Part model, mm, in its own coordinate system. Face numbers are marked on the shaded views. Give positions to 0.01 mm unless a question says otherwise; leave off trailing zeros. Order: outer loops, then holes, each group sorted by start corner. A loop starts at its lowest first (then second) coordinate and runs counter-clockwise, first axis right, second up. Notation, with made-up numbers: (20.25, -3.5) - (67.25, -3.5) arc R16 cw to (67.25, 3.5) - close; hole circle Ø1 at (82, 3). An arc over 180 degrees is marked (long way). One line per item, written item: value.
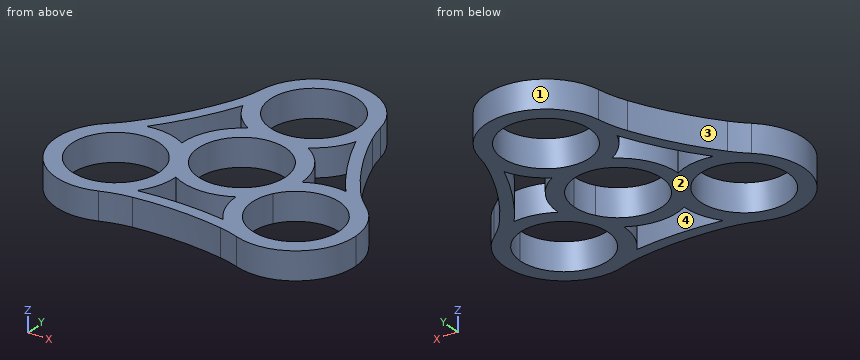
```python
from build123d import *

# Parameters (mm, degrees)
F1_DEPTH = 7
F2_R     = 30


with BuildPart() as f1:
    # F0 (on Top) → F1 (new body)
    with BuildSketch(Plane.XY):
        with BuildLine():
            ThreePointArc((-13.9458281821, 20.4760633317), (-11.3479038896, 16.1905618249), (-7.4833147735, 13))
            ThreePointArc((-7.4833147735, 13), (-3.8729833256, 14.4913767517), (4.26e-08, 15))
            ThreePointArc((4.26e-08, 15), (3.8729833668, 14.4913767407), (7.4833147735, 13))
            ThreePointArc((7.4833147735, 13), (11.4579364901, 16.3193134856), (14.0670033826, 20.7923694606))
            ThreePointArc((14.0670033826, 20.7923694606), (14.7649085798, 23.3547259819), (15, 26))
            ThreePointArc((15, 26), (14.9881318268, 26.5965771885), (14.9525460877, 27.1922103396))
            ThreePointArc((14.9525460877, 27.1922103396), (-0.6061990993, 40.9877457495), (-14.999987636, 25.9807406984))
            ThreePointArc((-14.999987636, 25.9807406984), (-14.7322921357, 23.1787292883), (-13.9458281821, 20.4760633317))
        make_face()
        with BuildLine():
            ThreePointArc((11, 26), (7.7781746081, 18.221825422), (4.26e-08, 15))
            ThreePointArc((4.26e-08, 15), (-7.7781746081, 33.778174578), (11, 26))
        make_face(mode=Mode.SUBTRACT)
        with BuildLine():
            ThreePointArc((-7.4833147735, 13), (-3.8729833208, 11.508623247), (5.26e-08, 11))
            ThreePointArc((5.26e-08, 11), (3.8729833716, 11.5086232606), (7.4833147735, 13))
            ThreePointArc((7.4833147735, 13), (3.8729833668, 14.4913767407), (4.26e-08, 15))
            ThreePointArc((4.26e-08, 15), (-3.8729833256, 14.4913767517), (-7.4833147735, 13))
        make_face()
        with BuildLine():
            ThreePointArc((5.26e-08, 11), (7.7781746116, 7.7781745745), (11, 0))
            ThreePointArc((11, 0), (10.6251840814, -2.8470095251), (9.5262794117, -5.5000000519))
            ThreePointArc((9.5262794117, -5.5000000519), (11.9032517523, -2.4002096819), (14.999987636, -0.0192593016))
            ThreePointArc((14.999987636, -0.0192593016), (14.999996909, -0.0096296528), (15, 0))
            ThreePointArc((15, 0), (12.9855635535, 7.5083379784), (7.4833147735, 13))
            ThreePointArc((7.4833147735, 13), (3.8729833716, 11.5086232606), (5.26e-08, 11))
        make_face()
        with BuildLine():
            ThreePointArc((15, 26), (14.7649085798, 23.3547259819), (14.0670033826, 20.7923694606))
            ThreePointArc((14.0670033826, 20.7923694606), (18.7632858244, 10.9661480048), (24.7057051058, 1.8394098167))
            ThreePointArc((24.7057051058, 1.8394098167), (27.439514459, 1.1691746013), (29.9999752719, 0))
            ThreePointArc((29.9999752719, 0), (21.1431293427, 12.8583865681), (14.9525460877, 27.1922103396))
            ThreePointArc((14.9525460877, 27.1922103396), (14.9881318268, 26.5965771885), (15, 26))
        make_face()
        with BuildLine():
            ThreePointArc((24.7057051058, 1.8394098167), (19.6953897867, 1.7322921357), (14.999987636, -0.0192593016))
            ThreePointArc((14.999987636, -0.0192593016), (14.4863920627, -3.8915864381), (12.9903810244, -7.5000000561))
            ThreePointArc((12.9903810244, -7.5000000561), (10.613408702, -10.5997903623), (7.5166728624, -12.9807406984))
            ThreePointArc((7.5166728624, -12.9807406984), (8.4039718058, -18.0825208181), (10.9732184665, -22.5785670147))
            ThreePointArc((10.9732184665, -22.5785670147), (13.3069353398, -24.8398041582), (16.0728718952, -26.545389933))
            ThreePointArc((16.0728718952, -26.545389933), (30.5273774124, -25.681814323), (37.5166604984, -13))
            ThreePointArc((37.5166604984, -13), (35.5022240519, -5.4916620216), (29.9999752719, 0))
            ThreePointArc((29.9999752719, 0), (27.439514459, 1.1691746013), (24.7057051058, 1.8394098167))
        make_face()
        with BuildLine():
            ThreePointArc((33.5166604984, -13), (19.6696510336, -23.6251840976), (12.9903810244, -7.5000000561))
            ThreePointArc((12.9903810244, -7.5000000561), (25.3636699632, -2.3748159024), (33.5166604984, -13))
        make_face(mode=Mode.SUBTRACT)
        with BuildLine():
            ThreePointArc((14.999987636, -0.0192593016), (11.9032517523, -2.4002096819), (9.5262794117, -5.5000000519))
            ThreePointArc((9.5262794117, -5.5000000519), (8.0302684195, -9.1084136221), (7.5166728624, -12.9807406984))
            ThreePointArc((7.5166728624, -12.9807406984), (10.613408702, -10.5997903623), (12.9903810244, -7.5000000561))
            ThreePointArc((12.9903810244, -7.5000000561), (14.4863920627, -3.8915864381), (14.999987636, -0.0192593016))
        make_face()
        with BuildLine():
            ThreePointArc((7.5166728624, -12.9807406984), (8.0302684195, -9.1084136221), (9.5262794117, -5.5000000519))
            ThreePointArc((9.5262794117, -5.5000000519), (-5.2e-09, -11), (-9.5262794169, -5.5000000429))
            ThreePointArc((-9.5262794169, -5.5000000429), (-8.0302684209, -9.1084136171), (-7.5166728624, -12.9807406984))
            ThreePointArc((-7.5166728624, -12.9807406984), (0, -15), (7.5166728624, -12.9807406984))
        make_face()
        with BuildLine():
            ThreePointArc((16.0728718952, -26.545389933), (13.3069353398, -24.8398041582), (10.9732184665, -22.5785670147))
            ThreePointArc((10.9732184665, -22.5785670147), (0.1153198416, -21.7325561849), (-10.7598769237, -22.3154731484))
            ThreePointArc((-10.7598769237, -22.3154731484), (-12.7072223233, -24.3479038896), (-14.999987636, -25.9807406984))
            ThreePointArc((-14.999987636, -25.9807406984), (0.5641247483, -24.7396804103), (16.0728718952, -26.545389933))
        make_face()
        with BuildLine():
            ThreePointArc((-7.5166604984, -13), (-7.5166635894, -12.9903703472), (-7.5166728624, -12.9807406984))
            ThreePointArc((-7.5166728624, -12.9807406984), (-10.6134087435, -10.5997903208), (-12.990381083, -7.4999999545))
            ThreePointArc((-12.990381083, -7.4999999545), (-14.4863920779, -3.8915863815), (-14.999987636, -0.0192593016))
            ThreePointArc((-14.999987636, -0.0192593016), (-19.8619082959, 1.7632073325), (-25.0402218491, 1.7861975541))
            ThreePointArc((-25.0402218491, 1.7861975541), (-28.1653690959, 0.8957580283), (-31.025417983, -0.6468204065))
            ThreePointArc((-31.025417983, -0.6468204065), (-35.1933295133, -21.0188566945), (-14.999987636, -25.9807406984))
            ThreePointArc((-14.999987636, -25.9807406984), (-12.7072223233, -24.3479038896), (-10.7598769237, -22.3154731484))
            ThreePointArc((-10.7598769237, -22.3154731484), (-8.3506491752, -17.9319492282), (-7.5166604984, -13))
        make_face()
        with BuildLine():
            ThreePointArc((-11.5166604984, -13), (-33.1418445808, -15.8470095215), (-12.990381083, -7.4999999545))
            ThreePointArc((-12.990381083, -7.4999999545), (-11.891476416, -10.1529904785), (-11.5166604984, -13))
        make_face(mode=Mode.SUBTRACT)
        with BuildLine():
            ThreePointArc((-7.5166728624, -12.9807406984), (-8.0302684209, -9.1084136171), (-9.5262794169, -5.5000000429))
            ThreePointArc((-9.5262794169, -5.5000000429), (-11.903251756, -2.4002096782), (-14.999987636, -0.0192593016))
            ThreePointArc((-14.999987636, -0.0192593016), (-14.4863920779, -3.8915863815), (-12.990381083, -7.4999999545))
            ThreePointArc((-12.990381083, -7.4999999545), (-10.6134087435, -10.5997903208), (-7.5166728624, -12.9807406984))
        make_face()
        with BuildLine():
            ThreePointArc((-9.5262794169, -5.5000000429), (-9.5262794409, 5.5000000013), (5.26e-08, 11))
            ThreePointArc((5.26e-08, 11), (-3.8729833208, 11.508623247), (-7.4833147735, 13))
            ThreePointArc((-7.4833147735, 13), (-12.9903810568, 7.5), (-14.999987636, -0.0192593016))
            ThreePointArc((-14.999987636, -0.0192593016), (-11.903251756, -2.4002096782), (-9.5262794169, -5.5000000429))
        make_face()
        with BuildLine():
            ThreePointArc((-25.0402218491, 1.7861975541), (-18.8786056661, 10.76640818), (-13.9458281821, 20.4760633317))
            ThreePointArc((-13.9458281821, 20.4760633317), (-14.7322921357, 23.1787292883), (-14.999987636, 25.9807406984))
            ThreePointArc((-14.999987636, 25.9807406984), (-21.707254091, 11.8812938422), (-31.025417983, -0.6468204065))
            ThreePointArc((-31.025417983, -0.6468204065), (-28.1653690959, 0.8957580283), (-25.0402218491, 1.7861975541))
        make_face()
    extrude(amount=F1_DEPTH)

    # F2
    f2_edges = [f1.edges().sort_by_distance(p)[0] for p in [
        (-14.999988, 25.980741, 3.5),
        (-31.025418, -0.64682, 3.5),
        (-14.999988, -25.980741, 3.5),
        (16.072872, -26.54539, 3.5),
        (14.952546, 27.19221, 3.5),
        (29.999975, 0, 3.5),
    ]]
    fillet(f2_edges, radius=F2_R)


solid = f1.part
```
1) Two-plate mould, pull along X, no slides. Class the marked faces 1, 2, 3 and 4: pulls with the +X half, pulls with the -X half, needs draft (parallel to the pull), parting line crosses it, or undercut.
Answer:
face 1: parting line crosses it
face 2: needs draft
face 3: pulls with the -X half
face 4: undercut
2) Drop flat-ended pins along their axis: P1, Ø6, axis at x = -29.5, y = -14, coming from the -Z side; P2, Ø1, axis at x = 22, z = 4.5, coming from the +Y side; P3, Ø1, axis at x = -20.5, z = 2.5, coming from the -Y side. Give the stop position or say it passes through.
Answer:
P1: passes through
P2: stops at y = 12.22
P3: stops at y = -27.92
3) Slice it at D-D on x = 0. Write the cut outline in (y, z), then the cut area to 3 significant figures.
Answer:
outline: (-24.73, 0) - (-21.73, 0) - (-21.73, 7) - (-24.73, 7) - close; (-15, 0) - (-11, 0) - (-11, 7) - (-15, 7) - close; (11, 0) - (15, 0) - (15, 7) - (11, 7) - close; (37, 0) - (41, 0) - (41, 7) - (37, 7) - close
area: 105 mm2
4) Slice it at C-C on y = 35.5. Write the cut outline in (x, z), then the cut area to 3 significant figures.
Answer:
outline: (-11.61, 0) - (-5.55, 0) - (-5.55, 7) - (-11.61, 7) - close; (5.55, 0) - (11.61, 0) - (11.61, 7) - (5.55, 7) - close
area: 84.9 mm2
5) Slice it at A-A on x = -18.5. Write the cut outline in (y, z), then the cut area to 3 significant figures.
Answer:
outline: (-27.45, 0) - (-23.24, 0) - (-23.24, 7) - (-27.45, 7) - close; (-2.76, 0) - (1.45, 0) - (1.45, 7) - (-2.76, 7) - close; (11.41, 0) - (17.75, 0) - (17.75, 7) - (11.41, 7) - close
area: 103 mm2
6) Wall check: line 1 along Y through (x, z) = (9.5, 0.75); line 2 along Y through (x, z) = (24, 6); line 3 along Y through (x, z) = (-1, 5). Give the ranges that are in metal, low to high. Write a range as [from, to].
Answer:
line 1: y = [-25.4, -22.38], [-20.45, -5.55], [5.55, 11.61], [14.39, 20.45], [31.55, 37.61]
line 2: y = [-27.93, -23.9], [-2.1, 1.93], [2.8, 8.09]
line 3: y = [-24.73, -21.73], [-14.97, -10.95], [10.95, 15.05], [36.95, 40.97]
7) Slice it at B-B on y = -19. Write the cut outline in (x, z), then the cut area to 3 significant figures.
Answer:
outline: (-36.26, 0) - (-31.74, 0) - (-31.74, 7) - (-36.26, 7) - close; (-13.3, 0) - (-8.77, 0) - (-8.77, 7) - (-13.3, 7) - close; (8.77, 0) - (13.3, 0) - (13.3, 7) - (8.77, 7) - close; (31.74, 0) - (36.26, 0) - (36.26, 7) - (31.74, 7) - close
area: 127 mm2
